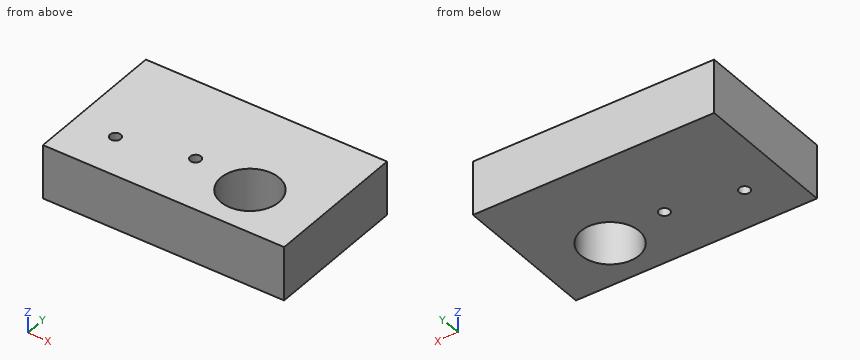
from build123d import *

# Parameters (mm, degrees)
F0_W     = 111.7238141596
F0_H     = 66.8160738423
F1_DEPTH = 25
F3_D     = 5
F5_D     = 5
F6_R     = 13.4792277867
F7_DEPTH = 25.001


with BuildPart() as f1:
    # F0 (on Top) → F1 (new body)
    with BuildSketch(Plane.XY):
        with Locations((-7.3526781052, 20.4115337692)):
            Rectangle(F0_W, F0_H)
    extrude(amount=F1_DEPTH)

    # F3 (through all)
    with Locations(Plane(origin=(0, 0, 0), x_dir=(1, 0, 0), z_dir=(0, 0, -1))):
        with Locations((-44.0534129739, -7.1848076768)):
            Hole(F3_D / 2)

    # F5 (through all)
    with Locations(Plane(origin=(0, 0, 0), x_dir=(1, 0, 0), z_dir=(0, 0, -1))):
        with Locations((-11.3455168903, -13.4060289711)):
            Hole(F5_D / 2)

    # F6 (on Top) → F7 (cut, through all)
    with BuildSketch(Plane.XY):
        with Locations((16.8637931347, 9.1420030221)):
            Circle(F6_R)
    extrude(amount=F7_DEPTH, mode=Mode.SUBTRACT)


solid = f1.part
Verification items for the finished model (mm, model axes). Coordinates: 2 decimals unless noted, no trailing zeros. Order: outer loops, then holes, each group sorted by start corner. A loop starts at its lowest first (then second) coordinate and runs counter-clockwise, first axis right, second up. Notation, with made-up numbers: M -27.75,-20 L 11.25,-20 A17 cw 11.25,4 Z; hole C 77.25,17.5 d3. An arc over 180 degrees is marked long. One line per item, written item: value. Start each with the question number.
Item 1: Sectioned sample at B-B on x = -11.5. Record the cut outline in (y, z), then the cut area to 3 significant figures.
Item 2: Sectioned sample at D-D on y = 12. Record the cut outline in (x, z).
Item 3: Depth check by flat-ended pin: P1, Ø24.5, axis at x = 16.86, y = 9.14, coming from the -Z side. Enter the tip coordinate at first touch or a pass-through.
Item 4: Sectioned sample at C-C on z = 3.75. Record the cut outline in (x, y).
Item 5: Sectioned sample at A-A on y = 20. Record the cut outline in (x, z), then the cut area to 3 significant figures.
Item 6: Thickness scan on probe 1 along X at (y, z) = (6, 22); probe 2 along X at (y, z) = (8, 17.75); probe 3 along Y at (x, z) = (26.5, 20). Record the ranges inside material, lowest first.
Calculated:
1. outline: M -13,0 L 10.91,0 L 10.91,25 L -13,25 Z; M 15.9,0 L 53.82,0 L 53.82,25 L 15.9,25 Z
1. area: 1,550 mm^2
2. outline: M -63.21,0 L -13.41,0 L -13.41,25 L -63.21,25 Z; M -9.28,0 L 3.69,0 L 3.69,25 L -9.28,25 Z; M 30.04,0 L 48.51,0 L 48.51,25 L 30.04,25 Z
3. P1: through
4. outline: M -63.21,-13 L 48.51,-13 L 48.51,53.82 L -63.21,53.82 Z; hole C -44.05,7.18 d5; hole C -11.35,13.41 d5; hole C 16.86,9.14 d26.96
5. outline: M -63.21,0 L 8.88,0 L 8.88,25 L -63.21,25 Z; M 24.85,0 L 48.51,0 L 48.51,25 L 24.85,25 Z
5. area: 2,390 mm^2
6. probe 1: -63.21 to -46.25, -41.85 to 3.76, 29.97 to 48.51
6. probe 2: -63.21 to -46.42, -41.69 to 3.43, 30.29 to 48.51
6. probe 3: -13 to -0.28, 18.57 to 53.82
